Geometry: final body of the model. Coordinates: model frame, mm. A direction names the side the tool comes from. Coordinates: 2 decimals unless noted, no trailing zeros. Loops run counter-clockwise (first coordinate to the right, second up) from the corner with the lowest first, then second, coordinate; pieces in that order, holes last. Notation, with made-up numbers: (6.5, 61) - (56.5, 61) arc R19 ccw to (56.5, 83) - close; hole circle Ø3 at (-18, 13). An arc over 180 degrees is marked (long way). Put each result on its own line as item: value. Start each with the question number.
1) Section B-B on x = 14. Output: boundary loops of the cut face in (y, z), and give its area (3 significant figures).
2) Section D-D on y = -15.5. Output: boundary loops of the cut face in (x, z).
3) Draft query along Z for faces 3 (the cylindrical face through (12.567, 13.243, 4.975)), 4 (the flat face through (-17, -8, 8)), 5 (the flat face through (23, 13.734, 4)). Return one class per face: +Z half, -Z half, draft (parallel to the pull), parting line (faces both ways), or undercut.
4) Section C-C on z = 6. Output: boundary loops of the cut face in (x, y).
5) Contact query for flat-ended pins moving along their axis: pin 1 Ø1.8 at (y, z) = (-26, 3) entering from -X; pin 2 Ø4 at (y, z) = (20, 5.5) entering from -X; pin 3 Ø1.1 at (x, z) = (23, 4.5) entering from +Y; pin 4 Ø18 at (x, y) = (0.19, -3.19) entering from -Z. Output: stop coordinate, or through.
6) Section A-A on y = -2.5. Output: boundary loops of the cut face in (x, z), and give its area (3 significant figures).
7) Reachability of faces 1 (the cylindrical face through (-12.59, 12.92, 4.89)), 2 (the flat face through (23, -20.266, 4)) from +Z, -Z, +X, -X, +Y, -Y: full face, straight path, thin tool, end or side. Return the list, or none.
8) Material intervals for line 1 along X through (y, z) = (19, 2); line 2 along Y through (x, z) = (3.5, 5.5); line 3 along X through (y, z) = (-20, 4.25), sorted ascending. Write a range as from..to.
Autodesk Inventor part; units mm, degrees
ref_plane "YZ Plane" through (0, 0, 0) normal (1, 0, 0) x (0, 1, 0)
ref_plane "XZ Plane" through (0, 0, 0) normal (0, 1, 0) x (-1, 0, 0)
ref_plane "XY Plane" through (0, 0, 0) normal (0, 0, 1) x (1, 0, 0)
sketch "Sketch1" plane through (0, 0, 0) normal (0, 0, 1) x (1, 0, 0)
  line L0 (21.5871, 13.6345) -> (17.0871, 18.1345)
  line L1 (17.0871, 18.1345) -> (-16.7129, 18.1345)
  line L2 (-16.7129, 18.1345) -> (-21.2129, 13.6345)
  line L3 (-21.0966, 13.6345) -> (-21.0966, -20.1655)
  line L4 (21.4709, -20.1655) -> (21.4709, 13.6345)
  line L5 (21.4709, -20.1655) -> (17.0871, -24.4078)
  line L6 (-16.7129, -24.4078) -> (17.0871, -24.4078)
  line L7 (-16.7129, -24.4078) -> (-21.0966, -20.1655)
  line L8 (-24.7129, -28.1655) -> (-24.7129, 13.6345) construction
  line L9 (25.0871, -28.1655) -> (-24.7129, -28.1655) construction
  line L10 (25.0871, -28.1655) -> (25.0871, 13.6345) construction
  line L11 (17.0871, 21.6345) -> (-16.7129, 21.6345) construction
  line L12 (-21.0552, -20.0655) -> (-16.6129, -24.5078)
  line L13 (-16.6129, -24.5078) -> (-16.6129, -28.1655)
  line L14 (-16.6129, -28.1655) -> (17.0871, -28.1655)
  line L15 (25.0871, -20.0655) -> (21.4295, -20.0655)
  line L16 (25.0871, 13.5345) -> (25.0871, -20.0655)
  line L17 (21.4295, 13.5345) -> (25.0871, 13.5345)
  line L18 (21.4295, 13.5345) -> (16.9871, 17.9768)
  line L19 (16.9871, 17.9768) -> (16.9871, 21.6345)
  line L20 (16.9871, 21.6345) -> (-16.6129, 21.6345)
  line L21 (-16.6129, 21.6345) -> (-16.6129, 17.9768)
  line L22 (-16.6129, 17.9768) -> (-21.0552, 13.5345)
  line L23 (-24.7129, 13.5345) -> (-21.0552, 13.5345)
  line L24 (-24.7129, -20.0655) -> (-24.7129, 13.5345)
  line L25 (-21.0552, -20.0655) -> (-24.7129, -20.0655)
  line L26 (-12.3129, -23.2655) -> (12.6871, -23.2655)
  line L27 (12.6871, -23.2655) -> (12.6871, 16.7345)
  line L28 (-12.3129, 16.7345) -> (12.6871, 16.7345)
  line L29 (-12.3129, -23.2655) -> (-12.3129, 16.7345)
  line L30 (14.6871, -25.2655) -> (-14.3129, -25.2655) construction
  line L31 (-14.3129, -25.2655) -> (-14.3129, 18.7345) construction
  line L32 (-14.3129, 18.7345) -> (14.6871, 18.7345) construction
  line L33 (14.6871, 18.7345) -> (14.6871, -25.2655) construction
  line L34 (-17.3129, 21.7345) -> (17.6871, 21.7345) construction
  line L35 (17.6871, 21.7345) -> (17.6871, -28.2655) construction
  line L36 (17.6871, -28.2655) -> (-17.3129, -28.2655) construction
  line L37 (-17.3129, -28.2655) -> (-17.3129, 21.7345) construction
  line L38 (-14.3129, -23.2655) -> (-14.3129, -25.2655)
  line L39 (-14.3129, -25.2655) -> (14.6871, -25.2655)
  line L40 (14.6871, -25.2655) -> (14.6871, -20.0655)
  line L41 (14.6871, -20.0655) -> (17.6871, -20.0655)
  line L42 (17.6871, -20.0655) -> (17.6871, 13.5345)
  line L43 (17.6871, 13.5345) -> (14.6871, 13.5345)
  line L44 (14.6871, 13.5345) -> (14.6871, 18.7345)
  line L45 (14.6871, 18.7345) -> (-14.3129, 18.7345)
  line L46 (-14.3129, 18.7345) -> (-14.3129, 13.5345)
  line L47 (-14.3129, 13.5345) -> (-17.3129, 13.5345)
  line L48 (-17.3129, 13.5345) -> (-17.3129, -20.0655)
  line L49 (-17.3129, -20.0655) -> (-14.3129, -20.0655)
  line L50 (-14.3129, -20.0655) -> (-14.3129, -23.2655)
  line L51 (-16.6129, -28.1655) -> (17.0871, -28.1655)
  line L52 (16.9871, -28.1655) -> (16.9871, -24.3509)
  line L53 (16.9871, -24.3509) -> (21.2726, -20.0655)
  line L54 (21.2726, -20.0655) -> (21.4295, -20.0655)
  point P0 (14.2, -44.8454)
  point P1 (16.9871, 19.8057)
  dimension "d74" = 2
  dimension "d75" = 5
  dimension "d76" = 135
extrude "Extrusion1" add sketch "Sketch1" along normal blind 8 contours L19 L18 L17 L4 L15 L54 L53 L52 L6 L40 L41 L42 L43 L44 L1 | L1 L44 L45 L46 L21 L20 L19 | L44 L43 L42 L41 L40 L6 L38 L50 L49 L48 L47 L46 L1 | L1 L46 L45 L44 | L46 L47 L48 L49 L50 L38 L6 L12 L25 L3 L23 L22 L21 L1 | L17 L16 L15 L4 | L3 L25 L24 L23 | L40 L39 L38 L6 | L6 L52 L14 L13 L12 L38 L39 L40 | L29 L28 L27 L26
sketch "Skizze7" plane through (0, 0, 8) normal (0, 0, 1) x (1, 0, 0)
  line L0 (-21.0552, -20.0655) -> (-16.6129, -24.5078)
  line L1 (-16.6129, -24.5078) -> (-16.6129, -28.1655)
  line L2 (-16.6129, -28.1655) -> (16.9871, -28.1655) construction
  line L3 (16.9871, -28.1655) -> (16.9871, -24.3509)
  line L4 (16.9871, -24.3509) -> (21.2726, -20.0655)
  line L5 (21.2726, -20.0655) -> (25.0871, -20.0655)
  line L6 (25.0871, -20.0655) -> (25.0871, 13.5345) construction
  line L7 (25.0871, 13.5345) -> (21.4295, 13.5345)
  line L8 (21.4295, 13.5345) -> (16.9871, 17.9768)
  line L9 (16.9871, 17.9768) -> (16.9871, 21.6345)
  line L10 (16.9871, 21.6345) -> (-16.6129, 21.6345) construction
  line L11 (-16.6129, 21.6345) -> (-16.6129, 17.9768)
  line L12 (-16.6129, 17.9768) -> (-21.0552, 13.5345)
  line L13 (-21.0552, 13.5345) -> (-24.7129, 13.5345)
  line L14 (-24.7129, 13.5345) -> (-24.7129, -20.0655) construction
  line L15 (-24.7129, -20.0655) -> (-21.0552, -20.0655)
  line L16 (-16.8129, 21.8345) -> (17.1871, 21.8345) construction
  line L17 (17.1871, 21.8345) -> (17.1871, 18.0597)
  line L18 (17.1871, 18.0597) -> (21.5123, 13.7345)
  line L19 (21.5123, 13.7345) -> (25.2871, 13.7345)
  line L20 (25.2871, 13.7345) -> (25.2871, -20.2655) construction
  line L21 (25.2871, -20.2655) -> (21.3554, -20.2655)
  line L22 (21.3554, -20.2655) -> (17.1871, -24.4338)
  line L23 (17.1871, -24.4338) -> (17.1871, -28.3655)
  line L24 (17.1871, -28.3655) -> (-16.8129, -28.3655) construction
  line L25 (-16.8129, -28.3655) -> (-16.8129, -24.5907)
  line L26 (-16.8129, -24.5907) -> (-21.1381, -20.2655)
  line L27 (-21.1381, -20.2655) -> (-24.9129, -20.2655)
  line L28 (-24.9129, -20.2655) -> (-24.9129, 13.7345) construction
  line L29 (-24.9129, 13.7345) -> (-21.1381, 13.7345)
  line L30 (-21.1381, 13.7345) -> (-16.8129, 18.0597)
  line L31 (-16.8129, 18.0597) -> (-16.8129, 21.8345)
  line L32 (-21.0552, 13.5345) -> (-24.7129, 13.5345)
  line L33 (-24.7129, 13.5345) -> (-24.7129, 13.7345)
  line L34 (-16.6129, 21.6345) -> (-16.6129, 17.9768)
  line L35 (-16.6129, 21.6345) -> (-16.8129, 21.6345)
  line L36 (25.0871, -20.0655) -> (25.0871, 13.5345)
  line L37 (25.0871, 13.5345) -> (25.0871, 13.7345)
  line L38 (16.9871, 21.6345) -> (17.1871, 21.6345)
  line L39 (16.9871, -28.1655) -> (17.1871, -28.1655)
  line L40 (25.0871, -20.0655) -> (25.0871, -20.2655)
  line L41 (-16.6129, -28.1655) -> (-16.8129, -28.1655)
  line L42 (-24.7129, -20.0655) -> (-24.7129, -20.2655)
  dimension "d94" = 0.2
extrude "IM_offset" add sketch "Skizze7" against normal up to surface (8 mm away)
sketch "Sketch8" plane through (-16.8129, 21.6345, 0) normal (0, 1, 0) x (1, 0, 0)
  line L0 (0, 0) -> (34, 0)
  line L1 (34, -8) -> (0, -8)
  line L2 (3.8129, -1.6478) -> (29.8129, -1.6478)
  arc A0 (3.8129, -1.6478) -> (29.8129, -1.6478) centre (16.8129, -1.6478) ccw
  line L3 (0, -8) -> (0, 0)
  line L4 (34, -8) -> (34, 0)
  point P0 (16.8129, 0)
  dimension "d86" = 26
  dimension "d88" = 0
extrude "Extrusion7" cut sketch "Sketch8" against normal blind 45 contours A0 L2 L1 | L1 A0
sketch "Sketch9" plane through (0, 0, 8) normal (0, 0, 1) x (1, 0, 0)
  line L0 (-11.3424, 21.6345) -> (-16.8129, 21.6345)
  line L1 (-24.7129, 13.7345) -> (-24.7129, -20.2655)
  line L2 (17.1871, -28.1655) -> (-16.8129, -28.1655)
  line L3 (25.0871, -20.0655) -> (25.0871, 13.7345)
  circle A0 centre (0.1871, -3.187) radius 27.0445
  circle A1 centre (0.1871, -3.187) radius 15
  line L4 (11.3424, 21.6345) -> (11.3424, -23.3655)
  line L5 (11.3424, -23.3655) -> (-11.3424, -23.3655)
  line L6 (-11.3424, -23.3655) -> (-11.3424, 21.6345)
  line L7 (17.1871, 21.6345) -> (11.3424, 21.6345)
  line L8 (-16.8129, 21.6345) -> (-16.8129, 18.0597)
  line L9 (-16.8129, 18.0597) -> (-21.1381, 13.7345)
  line L10 (-21.1381, 13.7345) -> (-24.7129, 13.7345)
  line L11 (17.1871, -28.1655) -> (17.1871, -24.4338)
  line L12 (17.1871, -24.4338) -> (21.3554, -20.2655)
  line L13 (21.3554, -20.2655) -> (25.0871, -20.2655)
  line L14 (25.0871, -20.2655) -> (25.0871, -20.0655)
  line L15 (25.0871, 13.7345) -> (21.5123, 13.7345)
  line L16 (21.5123, 13.7345) -> (17.1871, 18.0597)
  line L17 (17.1871, 18.0597) -> (17.1871, 21.6345)
  line L18 (-21.1381, -20.2655) -> (-24.7129, -20.2655)
  line L19 (-16.8129, -24.5907) -> (-21.1381, -20.2655)
  line L20 (-16.8129, -28.1655) -> (-16.8129, -24.5907)
  point P0 (0, 0)
  dimension "d91" = 30
extrude "Extrusion8" cut sketch "Sketch9" against normal through all contours L6 A1 | A1 L4 L6 | A1 L4
properties part number "20_Cube_Insert_Lens_Cylindrical_v3"
Answer block:
1. outline: (-28.17, 0) - (-9.04, 0) - (-9.04, 8) - (-28.17, 8) - close; (2.66, 0) - (21.63, 0) - (21.63, 8) - (2.66, 8) - close
1. area: 305 mm²
2. outline: (-24.71, 0) - (-8.38, 0) - (-8.38, 1.65) - (-13, 1.65) arc R13 cw to (-11.34, 8) - (-24.71, 8) - close; (8.75, 0) - (25.09, 0) - (25.09, 8) - (11.34, 8) arc R13 cw to (13, 1.65) - (8.75, 1.65) - close
3. face 3: undercut
3. face 4: +Z half
3. face 5: draft
4. outline: (-24.71, -20.27) - (-21.14, -20.27) - (-16.81, -24.59) - (-16.81, -28.17) - (17.19, -28.17) - (17.19, -24.43) - (21.36, -20.27) - (25.09, -20.27) - (25.09, 13.73) - (21.51, 13.73) - (17.19, 18.06) - (17.19, 21.63) - (12.25, 21.63) - (12.25, 5.73) arc R15 cw to (12.25, -12.1) - (12.25, -23.37) - (-12.25, -23.37) - (-12.25, -11.57) arc R15 cw to (-12.25, 5.2) - (-12.25, 21.63) - (-16.81, 21.63) - (-16.81, 18.06) - (-21.14, 13.73) - (-24.71, 13.73) - close
5. pin 1: stops at x = -16.81
5. pin 2: stops at x = -16.87
5. pin 3: stops at y = 13.73
5. pin 4: passes through
6. outline: (-24.71, 0) - (-14.8, 0) - (-14.8, 8) - (-24.71, 8) - close; (15.17, 0) - (25.09, 0) - (25.09, 8) - (15.17, 8) - close
6. area: 159 mm²
7. face 1: +Y
7. face 2: +Z, -Z, +X, -Y
8. line 1: x = -16.81..-13, 13..17.19
8. line 2: y = -28.17..-23.37
8. line 3: x = -24.71..-12.74, 12.74..25.09
